from build123d import *

# Parameters (mm, degrees)
SKETCH1_W                = 10
SKETCH1_H                = 15
BOSS_EXTRUDE1_DEPTH      = 115
SKETCH1_5_W              = 10
SKETCH1_5_H              = 15
CUT_EXTRUDE1_DEPTH       = 15
SKETCH6_W                = 15
SKETCH6_H                = 15
BOSS_EXTRUDE3_DEPTH      = 52.5
BOSS_EXTRUDE3_DEPTH_BACK = 67.5
CUT_EXTRUDE2_REACH       = 47
SKETCH7_W                = 35
SKETCH7_H                = 40
CUT_EXTRUDE3_DEPTH       = 15


with BuildPart() as part:
    # Sketch1 → Boss-Extrude1 (new body)
    with BuildSketch(Plane.XY):
        with BuildLine():
            Line((-10, 79.815551805), (-10, 94.815551805))
            ThreePointArc((-10, 94.815551805), (-39.085961763, 77.007283421), (-49.987139252, 44.691777486))
            Line((-49.987139252, 44.691777486), (20, 29.815551805))
            Line((20, 29.815551805), (20, 39.815551805))
            Line((20, 39.815551805), (0, 39.815551805))
            ThreePointArc((0, 39.815551805), (-7.071067812, 42.744483993), (-10, 49.815551805))
            Line((-10, 49.815551805), (-10, 64.815551805))
            Line((-10, 64.815551805), (-20, 64.815551805))
            Line((-20, 64.815551805), (-20, 79.815551805))
            Line((-20, 79.815551805), (-10, 79.815551805))
        make_face()
        with BuildLine():
            Line((20, 29.815551805), (-49.987139252, 44.691777486))
            ThreePointArc((-49.987139252, 44.691777486), (-41.519738184, 17.96698201), (-20, 0))
            Line((-20, 0), (-20, 24.815551805))
            Line((-20, 24.815551805), (20, 24.815551805))
            Line((20, 24.815551805), (20, 29.815551805))
        make_face()
        with Locations((-15, 72.315551805)):
            Rectangle(SKETCH1_W, SKETCH1_H)
    extrude(amount=-BOSS_EXTRUDE1_DEPTH)

    # Sketch1<5> → Cut-Extrude1 (cut)
    with BuildSketch(Plane.XY):
        with BuildLine():
            Line((-10, 79.815551805), (-10, 94.815551805))
            ThreePointArc((-10, 94.815551805), (-39.085961763, 77.007283421), (-49.987139252, 44.691777486))
            Line((-49.987139252, 44.691777486), (20, 29.815551805))
            Line((20, 29.815551805), (20, 39.815551805))
            Line((20, 39.815551805), (0, 39.815551805))
            ThreePointArc((0, 39.815551805), (-7.071067812, 42.744483993), (-10, 49.815551805))
            Line((-10, 49.815551805), (-10, 64.815551805))
            Line((-10, 64.815551805), (-20, 64.815551805))
            Line((-20, 64.815551805), (-20, 79.815551805))
            Line((-20, 79.815551805), (-10, 79.815551805))
        make_face()
        with Locations((-15, 72.315551805)):
            Rectangle(SKETCH1_5_W, SKETCH1_5_H)
    extrude(amount=-CUT_EXTRUDE1_DEPTH, mode=Mode.SUBTRACT)

    # Sketch6 → Boss-Extrude3 (add, two sides)
    with BuildSketch(Plane.XY.offset(-57.5)) as boss_extrude3_sk:
        with Locations((-12.5, 72.315551805)):
            Rectangle(SKETCH6_W, SKETCH6_H)
    extrude(amount=BOSS_EXTRUDE3_DEPTH)
    extrude(boss_extrude3_sk.sketch, amount=-BOSS_EXTRUDE3_DEPTH_BACK)

    # Sketch7 → Cut-Extrude2 (cut, up to next)
    with BuildSketch(Plane(origin=(-5, 0, 0), x_dir=(0, 0, -1), z_dir=(1, 0, 0)), mode=Mode.PRIVATE) as cut_extrude2_sk1:
        with Locations((62.5, 74.815551805)):
            Rectangle(SKETCH7_W, SKETCH7_H)
    cut_extrude2_tool1 = extrude(cut_extrude2_sk1.sketch, amount=-CUT_EXTRUDE2_REACH, mode=Mode.PRIVATE) & part.part
    add(cut_extrude2_tool1.solids().sort_by_distance((-5, 74.815552, -62.5))[0], mode=Mode.SUBTRACT)

    # Sketch8 → Cut-Extrude3 (cut)
    with BuildSketch(Plane(origin=(0, 39.815551805, 0), x_dir=(1, 0, 0), z_dir=(0, 1, 0))):
        with BuildLine():
            Line((5, 25), (5, 105))
            ThreePointArc((5, 105), (10, 110), (15, 105))
            Line((15, 105), (15, 25))
            ThreePointArc((15, 25), (10, 20), (5, 25))
        make_face()
    extrude(amount=-CUT_EXTRUDE3_DEPTH, mode=Mode.SUBTRACT)


solid = part.part
Geometry: final body of the model. Coordinates: model frame, mm. A direction names the side the tool comes from. Round coordinates to 2 decimals unless told otherwise and drop trailing zeros. Loops run counter-clockwise (first coordinate to the right, second up) from the corner with the lowest first, then second, coordinate; pieces in that order, holes last.
Q1. Pull-direction query (Z, two-part tool) for faces 6 (the flat face through (-23, 28, 0)), 7 (the flat face through (-29, 54.816, -62)), 8 (the flat face through (-10, 87, -30)); classes: released by +Z, released by -Z, zero draft, split by the parting line, or undercut.
Q2. Pin query (flat end, axial travel): P1, Ø1, axis at y = 47.5, z = -88.5, coming from the -X side; P2, Ø16.5, axis at y = 35.5, z = -51.5, coming from the -X side; P3, Ø10, axis at x = -24, z = -46, coming from the -Y side; P4, Ø6, axis at x = -22, y = 49, coming from the -Z side. Return the tip coordinate at first contact, or that it passes through.
Q3. Section B-B on y = 63. Return loops of the section in (x, z).
Q4. Section C-C on x = 10. Return loops of the section in (y, z).
Q5. Access query for faces 1 (the flat face through (-20, 72, -120)), 2 (the flat face through (-10, 87, -97)), 3 (the cylindrical face through (-6.993, 42.667, -64.3)), 4 (the flat face through (-20, 72, -10)), 5 (the flat face through (-5, 24.816, -57)). Directions: +Z, -Z, +X, -X, +Y, -Y. A direction counts if a zero-diameter tool reaches every point of the face in a straight line with its end or side. Return the directions, or none.
Q6. Section D-D on x = -38. Return loops of the section in (y, z), plus the area to 3 significant figures.
Q7. Section A-A on z = -62. Return loops of the section in (x, y), plus the area to 3 significant figures.
Q8. Material intervals for L1, parallel to X at y = 37, z = -80; L2, parallel to Z at x = -27, y = 35; L3, parallel to Z at x = -19, y = 82.5, sorted ascending.
Evaluation:
1. face 6: released by +Z
1. face 7: undercut
1. face 8: zero draft
2. P1: stops at x = -49.99
2. P2: stops at x = -49.96
2. P3: stops at y = 0
2. P4: stops at z = -115
3. outline: (-46.96, -115) - (-10, -115) - (-10, -80) - (-46.96, -80) - close; (-46.96, -45) - (-10, -45) - (-10, -15) - (-46.96, -15) - close
4. outline: (24.82, -115) - (39.82, -115) - (39.82, -110) - (24.82, -110) - close; (24.82, -20) - (39.82, -20) - (39.82, -15) - (31.94, -15) - (31.94, 0) - (24.82, 0) - close
5. face 1: -Z, -X, +Y, -Y
5. face 2: +Z, -Z, +X, +Y
5. face 3: +Z, -Z, +X
5. face 4: +Z, -X, +Y
5. face 5: +Z, -Z, +X, -Y
6. outline: (13.33, -115) - (78.32, -115) - (78.32, -80) - (54.82, -80) - (54.82, -45) - (78.32, -45) - (78.32, -15) - (42.14, -15) - (42.14, 0) - (13.33, 0) - close
6. area: 6,110 mm2
7. outline: (-49.19, 54.82) arc R50 ccw to (-20, 0) - (-20, 24.82) - (5, 24.82) - (5, 39.82) - (0, 39.82) arc R10 cw to (-10, 49.82) - (-10, 54.82) - close; (15, 24.82) - (20, 24.82) - (20, 39.82) - (15, 39.82) - close
7. area: 1,880 mm2
8. L1: x = -49.21 to 5, 15 to 20
8. L2: z = -115 to 0
8. L3: z = -115 to -80, -45 to -15
